Build history of the part. All positions in model axes, mm. A direction names the side the tool comes from. Give positions to 0.01 mm unless a question says otherwise; leave off trailing zeros. Order: outer loops, then holes, each group sorted by start corner. A loop starts at its lowest first (then second) coordinate and runs counter-clockwise, first axis right, second up. Notation, with made-up numbers: M 20.25,58 L 54.25,58 A15 ccw 54.25,82 Z; hole C 46,72 d4. An arc over 180 degrees is marked long. One line per item, written item: value.
Autodesk Inventor part; units mm, degrees
ref_plane "YZ Plane" through (0, 0, 0) normal (1, 0, 0) x (0, 1, 0)
ref_plane "XZ Plane" through (0, 0, 0) normal (0, 1, 0) x (-1, 0, 0)
ref_plane "XY Plane" through (0, 0, 0) normal (0, 0, 1) x (1, 0, 0)
sketch "Sketch1" plane through (0, 0, 0) normal (0, 1, 0) x (-1, 0, 0)
  point P0 (0, 0)
sketch "Sketch2" plane through (0, 0, 0) normal (0, 1, 0) x (-1, 0, 0)
  line L0 (0, 0) -> (-24.5, 0)
  line L1 (-24.5, 0) -> (-24.5, -15)
  line L2 (-24.5, -15) -> (0, -15)
  line L3 (0, -15) -> (0, 0)
  dimension "d0" = 24.5
  dimension "d1" = 15
extrude "Extrusion1" add sketch "Sketch2" along normal blind 6.5
sketch "Sketch3" plane through (0, 6.5, 0) normal (0, 1, 0) x (1, 0, 0)
  line L0 (0, 15) -> (0, 0)
  line L1 (24.5, 15) -> (0, 15)
  line L2 (0, 0) -> (2.5, 0)
  line L3 (2.5, 0) -> (2.5, 15)
  line L4 (2.5, 15) -> (0, 15)
  line L5 (0, 15) -> (0, 0)
  dimension "d4" = 2.5
extrude "Extrusion2" add sketch "Sketch3" along normal blind 8
fillet "Fillet1" radius 0.5 1 edges at (2.5, 6.5, -7.5)
properties part number "small_microswitch_holder"
1) Saw through at A-A, the plane z = -8. Write the cut outline in (x, y), then the cut area to 3 significant figures.
Check values:
outline: M 0,0 L 24.5,0 L 24.5,6.5 L 3,6.5 A0.5 cw 2.5,7 L 2.5,14.5 L 0,14.5 Z
area: 179 mm^2
2) Saw through at B-B, the plane y = 11.25. Write the cut outline in (x, z).
Check values:
outline: M 0,-15 L 2.5,-15 L 2.5,0 L 0,0 Z
3) Tool access for faces 1 (the face through (1, 14.5, -8)), 2 (the face through (2.5, 11, -7)): list every direction of +Z, -Z, +X, -X, +Y, -Y with a clear straight run to the whole face (end or side of a thin tool).
Check values:
face 1: +Z, -Z, +X, -X, +Y
face 2: +Z, -Z, +X, +Y
4) Drill centre lines: probe 1 along Y at (x, z) = (7.75, -12); probe 2 along X at (y, z) = (13, -13.5). Where is each one in solid material? Low to high. Write a range as from..to.
Check values:
probe 1: 0..6.5
probe 2: 0..2.5
5) Pin check, flat tips, straight feed: pin 1 (4.5 mm diameter, centred on x = 17.5, z = -5.5, fed in from +Y); pin 2 (4 mm diameter, centred on y = 11, z = -6.5, fed in from +X). Stop position of each tip, or through.
Check values:
pin 1: y = 6.5
pin 2: x = 2.5
6) Saw through at C-C, the plane x = 12. Write the cut outline in (y, z), then the cut area to 3 significant figures.
Check values:
outline: M 0,-15 L 6.5,-15 L 6.5,0 L 0,0 Z
area: 97.5 mm^2
